Geometry check sheet. Reference: drawing and pictorial views, mm from the part's lowest x, y, z. A direction names the side the tool comes from. Round coordinates to 2 decimals unless told otherwise and drop trailing zeros. Order: outer loops, then holes, each group sorted by start corner. A loop starts at its lowest first (then second) coordinate and runs counter-clockwise, first axis right, second up.
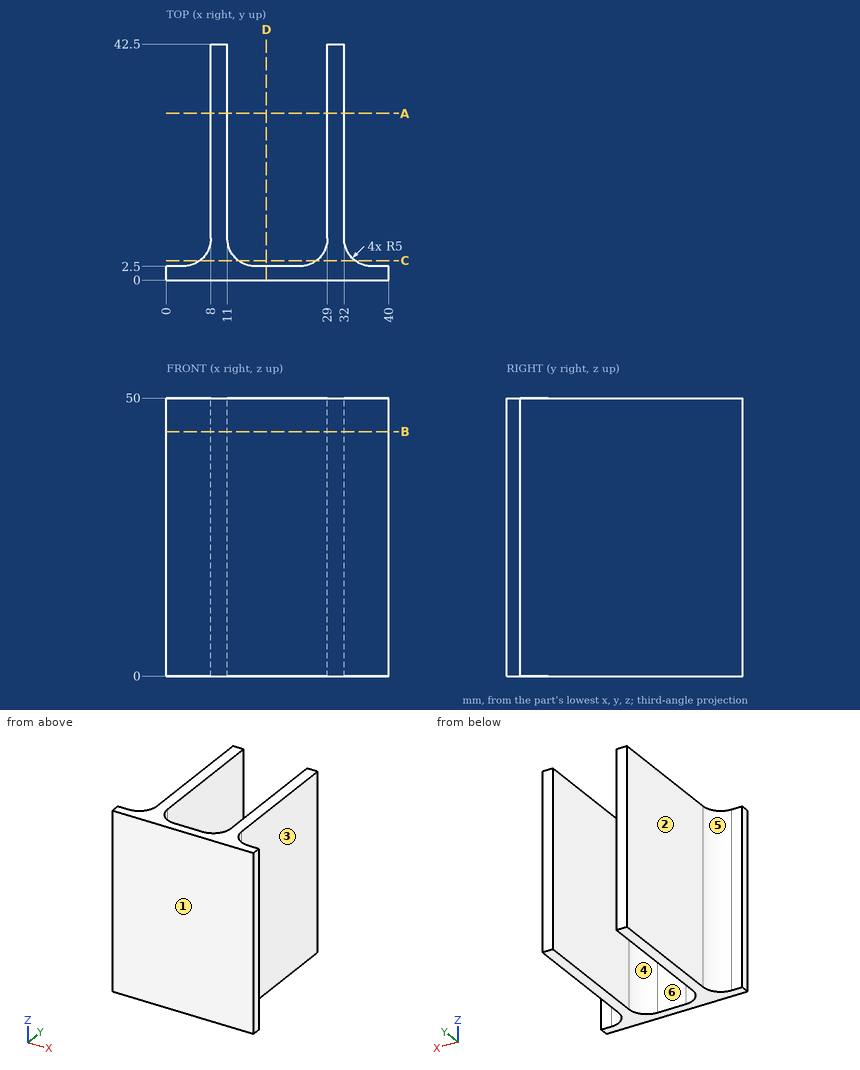
1) Go/stop test with flat-tipped pins: pin 1 Ø17.5 at (y, z) = (25.5, 12.5) entering from -X; pin 2 Ø12 at (x, y) = (33.5, 21.5) entering from +Z; pin 3 Ø6 at (y, z) = (9, 14.5) entering from -X; pin 4 Ø3.5 at (x, z) = (39, 21) entering from +Y. Record where each tip stops, or that it passes through.
2) Sectioned sample at D-D on x = 18. Record the cut outline in (y, z), then the cut area to 3 significant figures.
3) Tool access check on the marked faces 5 and 6. Record the directions out of +Z, -Z, +X, -X, +Y, -Y that give a thin tool (end or side, any length) a straight path to the whole face; none if there is none.
4) Scan lines: probe 1 along X at (y, z) = (32, 44); probe 2 along Y at (x, z) = (21.5, 30); probe 3 along Y at (x, z) = (11.5, 5). Record each from-to range of solid material in increasing order.
5) Sectioned sample at A-A on y = 30. Record the cut outline in (x, z), then the cut area to 3 significant figures.
6) Draft check along X on the marked faces 1, 2, 3 and 4. Enter one of: released by +X, released by -X, zero draft, split by the parting line, or undercut.
7) Sectioned sample at B-B on z = 44. Record the cut outline in (x, y), then the cut area to 3 significant figures.
8) Sectioned sample at C-C on y = 3.5. Record the cut outline in (x, z), then the cut area to 3 significant figures.
Returned:
1. pin 1: stops at x = 8
1. pin 2: stops at z = 50
1. pin 3: stops at x = 7.77
1. pin 4: stops at y = 2.5
2. outline: (0, 0) - (2.5, 0) - (2.5, 50) - (0, 50) - close
2. area: 125 mm2
3. face 5: +Z, -Z, -X, +Y
3. face 6: +Z, -Z, +Y
4. probe 1: x = 8 to 11, 29 to 32
4. probe 2: y = 0 to 2.5
4. probe 3: y = 0 to 5.32
5. outline: (8, 0) - (11, 0) - (11, 50) - (8, 50) - close; (29, 0) - (32, 0) - (32, 50) - (29, 50) - close
5. area: 300 mm2
6. face 1: zero draft
6. face 2: released by -X
6. face 3: released by +X
6. face 4: undercut
7. outline: (0, 0) - (40, 0) - (40, 2.5) - (37, 2.5) arc R5 cw to (32, 7.5) - (32, 42.5) - (29, 42.5) - (29, 7.5) arc R5 cw to (24, 2.5) - (16, 2.5) arc R5 cw to (11, 7.5) - (11, 42.5) - (8, 42.5) - (8, 7.5) arc R5 cw to (3, 2.5) - (0, 2.5) - close
7. area: 361 mm2
8. outline: (6, 0) - (13, 0) - (13, 50) - (6, 50) - close; (27, 0) - (34, 0) - (34, 50) - (27, 50) - close
8. area: 700 mm2
